Geometry check sheet. Reference: the model listing, model coordinates, mm. A direction names the side the tool comes from. Coordinates: 2 decimals unless noted, no trailing zeros. Order: outer loops, then holes, each group sorted by start corner. A loop starts at its lowest first (then second) coordinate and runs counter-clockwise, first axis right, second up. Notation, with made-up numbers: (75, 32.25) - (98, 32.25) arc R15 ccw to (98, 46.25) - close; hole circle Ø2 at (-40, 14). An arc over 180 degrees is marked (long way). Put each result on its own line as item: value.
from build123d import *

# Parameters (mm, degrees)
SKETCH1_W            = 6.266
SKETCH1_H            = 19.6
SKETCH1_R            = 1.475
SKETCH1_W_2          = 52.832
SKETCH1_H_2          = 5
BOSS_EXTRUDE2_DEPTH  = 3.2
SKETCH3_R            = 6.85
SKETCH3_R_2          = 4.85
BOSS_EXTRUDE3_DEPTH  = 5.975
SKETCH5_R            = 6.85
CUT_EXTRUDE2_DEPTH   = 2.4892
SKETCH10_R           = 6.846
BOSS_EXTRUDE10_DEPTH = 3.4858
SKETCH11_W           = 13.7
SKETCH11_H           = 5
BOSS_EXTRUDE11_DEPTH = 5.975
SKETCH15_W           = 52.832
SKETCH15_H           = 29.6
BOSS_EXTRUDE13_DEPTH = 3.2
SKETCH18_R           = 4.85
CUT_EXTRUDE9_DEPTH   = 32.638989886
SKETCH17_W           = 26.060927771
SKETCH17_H           = 40.585710908
CUT_EXTRUDE10_DEPTH  = 5.975
SKETCH12_W           = 52.832
SKETCH12_H           = 29.6
BOSS_EXTRUDE12_DEPTH = 3.2
SKETCH13_R           = 4.85
CUT_EXTRUDE3_DEPTH   = 10
SKETCH19_R           = 1.675
CUT_EXTRUDE11_DEPTH  = 3.2
SKETCH20_R           = 3.675
SKETCH20_R_2         = 1.675
BOSS_EXTRUDE14_DEPTH = 3.2
BOSS_EXTRUDE15_START = -3.2
SKETCH21_R           = 3.675
SKETCH21_R_2         = 1.675
BOSS_EXTRUDE15_DEPTH = 3.2
SKETCH27_R           = 4.85
CUT_EXTRUDE18_DEPTH  = 188
SKETCH30_R           = 6.85
SKETCH30_R_2         = 4.85
BOSS_EXTRUDE17_DEPTH = 3.2
BOSS_EXTRUDE18_DEPTH = 3.2
SKETCH32_R           = 6.425
CUT_EXTRUDE19_DEPTH  = 1.6


with BuildPart() as part:
    # Sketch1 → Boss-Extrude2 (new body)
    # profile 1 of 4: a face of its own
    with BuildSketch(Plane.XY):
        with Locations((-23.283, 0)):
            Rectangle(SKETCH1_W, SKETCH1_H)
        with Locations((-23.95, -4.974)):
            Circle(SKETCH1_R, mode=Mode.SUBTRACT)
        with Locations((-23.95, 4.974)):
            Circle(SKETCH1_R, mode=Mode.SUBTRACT)
    # profile 2 of 4: a face of its own
    with BuildSketch(Plane.XY):
        with Locations((23.283, 0)):
            Rectangle(SKETCH1_W, SKETCH1_H)
        with Locations((23.95, -4.974)):
            Circle(SKETCH1_R, mode=Mode.SUBTRACT)
        with Locations((23.95, 4.974)):
            Circle(SKETCH1_R, mode=Mode.SUBTRACT)
    # profile 3 of 4: a face of its own
    with BuildSketch(Plane.XY):
        with Locations((0, 12.3)):
            Rectangle(SKETCH1_W_2, SKETCH1_H_2)
    # profile 4 of 4: a face of its own
    with BuildSketch(Plane.XY):
        with Locations((0, -12.3)):
            Rectangle(SKETCH1_W_2, SKETCH1_H_2)
    extrude(amount=BOSS_EXTRUDE2_DEPTH)



with BuildPart() as body_2:
    # Sketch3 → Boss-Extrude3 (new body)
    with BuildSketch(Plane(origin=(0, 0, 0), x_dir=(-1, 0, 0), z_dir=(0, 0, -1))):
        with Locations(Location((10.076, 0.11, 0), (0, 0, 180))):
            Circle(SKETCH3_R)
        with Locations(Location((10.076, 0.11, 0), (0, 0, 180))):
            Circle(SKETCH3_R_2, mode=Mode.SUBTRACT)
    extrude(amount=BOSS_EXTRUDE3_DEPTH)

    # Sketch5 → Cut-Extrude2 (cut)
    with BuildSketch(Plane.XY):
        with Locations((-10.076, 0.11)):
            Circle(SKETCH5_R)
    extrude(amount=-CUT_EXTRUDE2_DEPTH, mode=Mode.SUBTRACT)

    # Sketch10 → Boss-Extrude10 (add)
    with BuildSketch(Plane(origin=(0, 0, -5.975), x_dir=(-1, 0, 0), z_dir=(0, 0, -1))):
        Polygon((16.93, -14.8), (16.93, 14.8), (3.23, 14.8), (3.23, 0.11), (3.23, -14.8), align=None)
        with Locations((10.076, 0.11)):
            Circle(SKETCH10_R, mode=Mode.SUBTRACT)
    extrude(amount=-BOSS_EXTRUDE10_DEPTH)


with BuildPart() as boss_extrude10_kept_piece:
    # of the separate pieces the step leaves, the one the design keeps (boss_extrude10_pieces_kept)
    add(body_2.part.solids().sort_by_distance((-3.23, -0.124059821, -5.975))[0])


with BuildPart() as part_1:
    add(part.part)

    add(boss_extrude10_kept_piece.part)  # Boss-Extrude11 merges Boss-Extrude10 kept piece
    # Sketch11 → Boss-Extrude11 (add)
    with BuildSketch(Plane(origin=(0, 0, -5.975), x_dir=(-1, 0, 0), z_dir=(0, 0, -1))):
        with Locations((10.08, 12.3)):
            Rectangle(SKETCH11_W, SKETCH11_H)
        with Locations((10.08, -12.3)):
            Rectangle(SKETCH11_W, SKETCH11_H)
    extrude(amount=-BOSS_EXTRUDE11_DEPTH)

    # Sketch15 → Boss-Extrude13 (add)
    with BuildSketch(Plane(origin=(0, 0, 0), x_dir=(-1, 0, 0), z_dir=(0, 0, -1))):
        Rectangle(SKETCH15_W, SKETCH15_H)
    extrude(amount=-BOSS_EXTRUDE13_DEPTH)

    # Sketch18 → Cut-Extrude9 (cut, through all)
    with BuildSketch(Plane(origin=(0, 0, -5.975), x_dir=(-1, 0, 0), z_dir=(0, 0, -1))):
        with Locations(Location((10.076, 0.11, 0), (0, 0, 180))):
            Circle(SKETCH18_R)
    extrude(amount=-CUT_EXTRUDE9_DEPTH, mode=Mode.SUBTRACT)

    # Sketch17 → Cut-Extrude10 (cut)
    with BuildSketch(Plane(origin=(0, 0, -5.975), x_dir=(-1, 0, 0), z_dir=(0, 0, -1))):
        with Locations((8.607278897, -0.029886385)):
            Rectangle(SKETCH17_W, SKETCH17_H)
    extrude(amount=-CUT_EXTRUDE10_DEPTH, mode=Mode.SUBTRACT)

    # Sketch12 → Boss-Extrude12 (add)
    with BuildSketch(Plane.XY.offset(3.2)):
        Rectangle(SKETCH12_W, SKETCH12_H)
    extrude(amount=-BOSS_EXTRUDE12_DEPTH)

    # Sketch13 → Cut-Extrude3 (cut)
    with BuildSketch(Plane(origin=(0, 0, 0), x_dir=(-1, 0, 0), z_dir=(0, 0, -1))):
        with Locations((10.076, 0.11)):
            Circle(SKETCH13_R)
    extrude(amount=-CUT_EXTRUDE3_DEPTH, mode=Mode.SUBTRACT)

    # Sketch19 → Cut-Extrude11 (cut)
    with BuildSketch(Plane.XY.offset(3.2)):
        with Locations((0, -13.025)):
            Circle(SKETCH19_R)
        with Locations((-23.741, 13.587)):
            Circle(SKETCH19_R)
        with Locations((23.741, 13.587)):
            Circle(SKETCH19_R)
    extrude(amount=-CUT_EXTRUDE11_DEPTH, mode=Mode.SUBTRACT)

    # Sketch20 → Boss-Extrude14 (add)
    with BuildSketch(Plane.XY.offset(3.2)):
        with Locations((0, -13.025)):
            Circle(SKETCH20_R)
        with Locations((0, -13.025)):
            Circle(SKETCH20_R_2, mode=Mode.SUBTRACT)
    extrude(amount=-BOSS_EXTRUDE14_DEPTH)

    # Sketch21 → Boss-Extrude15 (add)
    # profile 1 of 2: a face of its own
    with BuildSketch(Plane(origin=(0, 0, 0), x_dir=(-1, 0, 0), z_dir=(0, 0, -1)).offset(BOSS_EXTRUDE15_START)):
        with Locations((23.741, 13.587)):
            Circle(SKETCH21_R)
        with Locations(Location((23.741, 13.587, 0), (0, 0, 180))):
            Circle(SKETCH21_R_2, mode=Mode.SUBTRACT)
    # profile 2 of 2: a face of its own
    with BuildSketch(Plane(origin=(0, 0, 0), x_dir=(-1, 0, 0), z_dir=(0, 0, -1)).offset(BOSS_EXTRUDE15_START)):
        with Locations((-23.741, 13.587)):
            Circle(SKETCH21_R)
        with Locations(Location((-23.741, 13.587, 0), (0, 0, 180))):
            Circle(SKETCH21_R_2, mode=Mode.SUBTRACT)
    extrude(amount=BOSS_EXTRUDE15_DEPTH)

    # Sketch27 → Cut-Extrude18 (cut)
    with BuildSketch(Plane.XY.offset(3.2)):
        with Locations((11.074, 0)):
            Circle(SKETCH27_R)
    extrude(amount=-CUT_EXTRUDE18_DEPTH, mode=Mode.SUBTRACT)

    # Sketch30 → Boss-Extrude17 (add)
    # profile 1 of 2: a face of its own
    with BuildSketch(Plane.XY.offset(3.2)):
        with Locations((0, 22.8)):
            Circle(SKETCH30_R)
        with Locations((0, 22.8)):
            Circle(SKETCH30_R_2, mode=Mode.SUBTRACT)
    # profile 2 of 2: a face of its own
    with BuildSketch(Plane.XY.offset(3.2)):
        with BuildLine():
            ThreePointArc((6.85, 22.8), (0, 15.95), (-6.85, 22.8))
            Line((-6.85, 22.8), (-6.85, 14.8))
            Line((-6.85, 14.8), (6.85, 14.8))
            Line((6.85, 14.8), (6.85, 22.8))
        make_face()
    extrude(amount=-BOSS_EXTRUDE17_DEPTH)

    # Sketch31 → Boss-Extrude18 (add)
    with BuildSketch(Plane.XY.offset(3.2)):
        with BuildLine():
            Line((-6.85, 14.8), (-6.85, 22.8))
            ThreePointArc((-6.85, 22.8), (-6.602617872, 24.624263479), (-5.878339492, 26.316763401))
            ThreePointArc((-5.878339492, 26.316763401), (-9.334173967, 20.802087814), (-11.85, 14.8))
            Line((-11.85, 14.8), (-6.85, 14.8))
        make_face()
        with BuildLine():
            ThreePointArc((5.878339492, 26.316763401), (6.602617872, 24.624263479), (6.85, 22.8))
            Line((6.85, 22.8), (6.85, 14.8))
            Line((6.85, 14.8), (11.85, 14.8))
            ThreePointArc((11.85, 14.8), (9.334173967, 20.802087814), (5.878339492, 26.316763401))
        make_face()
    extrude(amount=-BOSS_EXTRUDE18_DEPTH)

    # Sketch32 → Cut-Extrude19 (cut)
    with BuildSketch(Plane.XY.offset(3.2)):
        with Locations((-10.076, 0.11)):
            Circle(SKETCH32_R)
        with Locations((11.074, 0)):
            Circle(SKETCH32_R)
    extrude(amount=-CUT_EXTRUDE19_DEPTH, mode=Mode.SUBTRACT)


solid = part_1.part
Q1. Depth check by flat-ended pin: pin 1 Ø1 at (y, z) = (-9, 1) entering from +X; pin 2 Ø1.6 at (x, z) = (-11, 1.5) entering from -Y; pin 3 Ø1 at (x, z) = (18, 1) entering from +Y. Enter the tip coordinate at first touch or a pass-through.
Answer block:
pin 1: stops at x = 26.42
pin 2: stops at y = -14.8
pin 3: stops at y = 14.8
Q2. Section check D-D on y = 22.8. Record the boundary of the cut face in (x, z), then the cut area to 3 significant figures.
Answer block:
outline: (-8.22, 0) - (-4.85, 0) - (-4.85, 3.2) - (-8.22, 3.2) - close; (4.85, 0) - (8.22, 0) - (8.22, 3.2) - (4.85, 3.2) - close
area: 21.6 mm^2
Q3. Section check B-B on y = 13. Record the boundary of the cut face in (x, z).
Answer block:
outline: (-27.37, 0) - (-25.31, 0) - (-25.31, 3.2) - (-27.37, 3.2) - close; (-22.17, 0) - (22.17, 0) - (22.17, 3.2) - (-22.17, 3.2) - close; (25.31, 0) - (27.37, 0) - (27.37, 3.2) - (25.31, 3.2) - close
Q4. Access from +Z, -Z, +X, -X, +Y, -Y to the whole of each face (thin tool, end or side, straight path). Record for faces 1 (the flat face through (12, 5, 1.6)), 2 (the flat face through (26.416, -2, 2)), 3 (the flat face through (-15, -14.8, 2)), 4 (the flat face through (-16, 14.8, 2)).
Answer block:
face 1: +Z
face 2: +Z, -Z, +X, -Y
face 3: +Z, -Z, -X, -Y
face 4: +Z, -Z, +Y
Q5. Section check C-C on x = 13. Record the boundary of the cut face in (y, z).
Answer block:
outline: (-14.8, 0) - (-4.45, 0) - (-4.45, 1.6) - (-6.13, 1.6) - (-6.13, 3.2) - (-14.8, 3.2) - close; (4.45, 0) - (14.8, 0) - (14.8, 3.2) - (6.13, 3.2) - (6.13, 1.6) - (4.45, 1.6) - close
Q6. Section check A-A on x = 0. Record the boundary of the cut face in (y, z).
Answer block:
outline: (-16.7, 0) - (-14.7, 0) - (-14.7, 3.2) - (-16.7, 3.2) - close; (-11.35, 0) - (17.95, 0) - (17.95, 3.2) - (-11.35, 3.2) - close; (27.65, 0) - (29.65, 0) - (29.65, 3.2) - (27.65, 3.2) - close
Q7. Thickness scan on L1, parallel to Y at x = 0, z = 2.35; L2, parallel to X at y = -1, z = 2.1; L3, parallel to Y at x = 5.5, z = 2.25. Record the ranges inside material, lowest first. Write a range as [from, to].
Answer block:
L1: y = [-16.7, -14.7], [-11.35, 17.95], [27.65, 29.65]
L2: x = [-26.42, -16.4], [-3.75, 4.73], [17.42, 26.42]
L3: y = [-14.8, -3.2], [3.2, 26.88]
Q8. Draft check along X on faces 5 (the cylindrical face through (-3.948, 2.04, 2.411)), 6 (the flat face through (-26.416, -2, 2)), 7 (the flat face through (0, 2, 0)). Enter one of: pulls with the +X half, pulls with the -X half, needs draft (parallel to the pull), parting line crosses it, or undercut.
Answer block:
face 5: undercut
face 6: pulls with the -X half
face 7: needs draft
